Here's how the part is built. I have some questions about the finished solid (model axes, mm). Give positions to 0.01 mm unless a question says otherwise; leave off trailing zeros. Write each loop counter-clockwise with the first axis right and the second up, starting at its lowest first coordinate (ties: lowest second). Pieces come first, ordered by that corner, then holes. Notation, with made-up numbers: (-8.75, 67.25) -> (9.25, 67.25) arc R16 cw to (9.25, 80.25) -> close; hole circle Ø7 at (36.5, -1). An arc over 180 degrees is marked (long way). Answer as CSV lines item,"result". Start each with the question number.
from build123d import *

# Parameters (mm, degrees)
REVOLVE1_ANGLE                 = 180
SKETCH2_W                      = 20
SKETCH2_H                      = 45
CUT_EXTRUDE1_DEPTH             = 35.641016151
CBORE_FOR_M3_SHCS1_D           = 3.4
CBORE_FOR_M3_SHCS1_CBORE_D     = 6.5
CBORE_FOR_M3_SHCS1_CBORE_DEPTH = 4


with BuildPart() as part:
    # Sketch1 → Revolve1 (revolve)
    with BuildSketch(Plane(origin=(0, 0, 0), x_dir=(1, 0, 0), z_dir=(0, 1, 0))):
        with BuildLine():
            Line((20, 0), (-20, 0))
            ThreePointArc((-20, 0), (0, 20), (20, 0))
        make_face()
    revolve(axis=Axis((20, 0, 0), (-1, 0, 0)), revolution_arc=REVOLVE1_ANGLE)

    # Sketch2 → Cut-Extrude1 (cut, through all)
    with BuildSketch(Plane(origin=(0, 0, 0), x_dir=(1, 0, 0), z_dir=(0, 1, 0))):
        with Locations((-20, 0)):
            Rectangle(SKETCH2_W, SKETCH2_H)
        with Locations((20, 0)):
            Rectangle(SKETCH2_W, SKETCH2_H)
    extrude(amount=-CUT_EXTRUDE1_DEPTH, mode=Mode.SUBTRACT)

    # CBORE for M3 SHCS1 (through all)
    with Locations(Plane(origin=(0, -20, 0), x_dir=(0, 0, -1), z_dir=(0, -1, 0))):
        with Locations((0, 0)):
            CounterBoreHole(CBORE_FOR_M3_SHCS1_D / 2, CBORE_FOR_M3_SHCS1_CBORE_D / 2, CBORE_FOR_M3_SHCS1_CBORE_DEPTH)


solid = part.part
Item 1: If we section it at B-B (x = 0): Please give me the cut outline in (y, z).
Item 2: If we section it at D-D (y = -5): Please give me the cut outline in (x, z).
Item 3: If we section it at A-A (z = 0): Please give me the cut outline in (x, y).
Item 4: If I drill on line 1 (X direction, y = -6.5, z = 0); line 2 (X direction, y = -17.45, z = 0); line 3 (Y direction, x = -1.25, z = 2.5), over which ranges is the centre line in solid material (lowest first)? Write a range as [from, to].
Item 5: I'm going to push flat-ended pins straight in: pin 1 (4 mm diameter, centred on x = 5.5, z = -2, fed in from -Y); pin 2 (5 mm diameter, centred on x = 3.5, y = -15, fed in from -Z); pin 3 (10 mm diameter, centred on x = -6.5, y = -10, fed in from +Z). Where does each tip first touch, or does it pass through?
Item 6: If we section it at C-C (y = -12.25): Please give me the cut outline in (x, z), and give its area (3 significant figures).
Item 7: We'd pull the mould along X, two halves only. Please class faces 1 (the face through (-1.978, -17.893, 2.579)), 2 (the face through (-2, 0, 0)), 3 (the face through (-1.4, -16, -1.4)), 4 (the face through (10, -7, 0)): released by +X, released by -X, zero draft, split by the parting line, or undercut.
Final values:
1,outline,"(-19.73, -3.25) arc R20 ccw to (0, -20) -> (0, -1.7) -> (-16, -1.7) -> (-16, -3.25) -> close; (-19.73, 3.25) -> (-16, 3.25) -> (-16, 1.7) -> (0, 1.7) -> (0, 20) arc R20 ccw to start"
2,outline,"(-10, -16.58) arc R19.36 ccw to (10, -16.58) -> (10, 16.58) arc R19.36 ccw to (-10, 16.58) -> close; hole circle Ø3.4 at (0, 0)"
3,outline,"(-10, -17.32) arc R20 ccw to (-3.25, -19.73) -> (-3.25, -16) -> (-1.7, -16) -> (-1.7, 0) -> (-10, 0) -> close; (1.7, -16) -> (3.25, -16) -> (3.25, -19.73) arc R20 ccw to (10, -17.32) -> (10, 0) -> (1.7, 0) -> close"
4,line 1,"[-10, -1.7], [1.7, 10]"
4,line 2,"[-9.77, -3.25], [3.25, 9.77]"
4,line 3,"[-16, 0]"
5,pin 1,"y = -19.63"
5,pin 2,"z = -15.28"
5,pin 3,"z = 18.76"
6,outline,"(-10, -12.24) arc R15.81 ccw to (10, -12.24) -> (10, 12.24) arc R15.81 ccw to (-10, 12.24) -> close; hole circle Ø3.4 at (0, 0)"
6,area,"578 mm2"
7,face 1,"undercut"
7,face 2,"zero draft"
7,face 3,"undercut"
7,face 4,"released by +X"
